```python
from build123d import *

# Parameters (mm, degrees)
F0_W     = 76
F0_H     = 46
F0_R     = 2.7
F1_DEPTH = 2
F2_R     = 6
F5_DEPTH = 25


with BuildPart() as f1:
    # F0 (on Top) → F1 (new body)
    with BuildSketch(Plane.XY):
        with Locations((-38, 0)):
            Rectangle(F0_W, F0_H)
        Polygon((-71.8, 11.2694276696), (-71.8, 15.2), (-61.6, 15.2), (-51.4, 15.2), (-51.4, 11.2694276696), (-51.4, -11.2694276696), (-51.4, -15.2), (-61.6, -15.2), (-71.8, -15.2), (-71.8, -11.2694276696), align=None, mode=Mode.SUBTRACT)
        Polygon((-50.6, 11.2694276696), (-50.6, 15.2), (-40.4, 15.2), (-30.2, 15.2), (-30.2, 11.2694276696), (-30.2, -11.2694276696), (-30.2, -15.2), (-40.4, -15.2), (-50.6, -15.2), (-50.6, -11.2694276696), align=None, mode=Mode.SUBTRACT)
        with Locations((-25.5, -6)):
            Circle(F0_R, mode=Mode.SUBTRACT)
        Polygon((-10.6, 15.2), (-0.4, 15.2), (-0.4, 11.2694276696), (-0.4, -11.2694276696), (-0.4, -15.2), (-10.6, -15.2), (-20.8, -15.2), (-20.8, -11.2694276696), (-20.8, 11.2694276696), (-20.8, 15.2), align=None, mode=Mode.SUBTRACT)
        with Locations((-25.5, 6)):
            Circle(F0_R, mode=Mode.SUBTRACT)
        with BuildLine():
            Line((-61.6, 15.2), (-71.8, 15.2))
            Line((-71.8, 15.2), (-71.8, 11.2694276696))
            ThreePointArc((-71.8, 11.2694276696), (-67.0655603291, 14.1833582162), (-61.6, 15.2))
        make_face()
        with BuildLine():
            Line((-51.4, 15.2), (-61.6, 15.2))
            ThreePointArc((-61.6, 15.2), (-56.1344396709, 14.1833582162), (-51.4, 11.2694276696))
            Line((-51.4, 11.2694276696), (-51.4, 15.2))
        make_face()
        with BuildLine():
            Line((-51.4, -15.2), (-51.4, -11.2694276696))
            ThreePointArc((-51.4, -11.2694276696), (-56.1344396709, -14.1833582162), (-61.6, -15.2))
            Line((-61.6, -15.2), (-51.4, -15.2))
        make_face()
        with BuildLine():
            ThreePointArc((-61.6, -15.2), (-67.0655603291, -14.1833582162), (-71.8, -11.2694276696))
            Line((-71.8, -11.2694276696), (-71.8, -15.2))
            Line((-71.8, -15.2), (-61.6, -15.2))
        make_face()
        with BuildLine():
            Line((-40.4, 15.2), (-50.6, 15.2))
            Line((-50.6, 15.2), (-50.6, 11.2694276696))
            ThreePointArc((-50.6, 11.2694276696), (-45.8655603291, 14.1833582162), (-40.4, 15.2))
        make_face()
        with BuildLine():
            Line((-30.2, 15.2), (-40.4, 15.2))
            ThreePointArc((-40.4, 15.2), (-34.9344396709, 14.1833582162), (-30.2, 11.2694276696))
            Line((-30.2, 11.2694276696), (-30.2, 15.2))
        make_face()
        with BuildLine():
            ThreePointArc((-20.8, 11.2694276696), (-16.0655603291, 14.1833582162), (-10.6, 15.2))
            Line((-10.6, 15.2), (-20.8, 15.2))
            Line((-20.8, 15.2), (-20.8, 11.2694276696))
        make_face()
        with BuildLine():
            Line((-0.4, 11.2694276696), (-0.4, 15.2))
            Line((-0.4, 15.2), (-10.6, 15.2))
            ThreePointArc((-10.6, 15.2), (-5.1344396709, 14.1833582162), (-0.4, 11.2694276696))
        make_face()
        with BuildLine():
            Line((-0.4, -15.2), (-0.4, -11.2694276696))
            ThreePointArc((-0.4, -11.2694276696), (-5.1344396709, -14.1833582162), (-10.6, -15.2))
            Line((-10.6, -15.2), (-0.4, -15.2))
        make_face()
        with BuildLine():
            ThreePointArc((-10.6, -15.2), (-16.0655603291, -14.1833582162), (-20.8, -11.2694276696))
            Line((-20.8, -11.2694276696), (-20.8, -15.2))
            Line((-20.8, -15.2), (-10.6, -15.2))
        make_face()
        with BuildLine():
            Line((-30.2, -15.2), (-30.2, -11.2694276696))
            ThreePointArc((-30.2, -11.2694276696), (-34.9344396709, -14.1833582162), (-40.4, -15.2))
            Line((-40.4, -15.2), (-30.2, -15.2))
        make_face()
        with BuildLine():
            ThreePointArc((-40.4, -15.2), (-45.8655603291, -14.1833582162), (-50.6, -11.2694276696))
            Line((-50.6, -11.2694276696), (-50.6, -15.2))
            Line((-50.6, -15.2), (-40.4, -15.2))
        make_face()
    extrude(amount=F1_DEPTH)

    # F2
    f2_edges = [f1.edges().sort_by_distance(p)[0] for p in [
        (-71.8, 11.269428, 1),
        (-71.8, -11.269428, 1),
        (-51.4, -11.269428, 1),
        (-51.4, 11.269428, 1),
        (-50.6, 11.269428, 1),
        (-50.6, -11.269428, 1),
        (-20.8, 11.269428, 1),
        (-20.8, -11.269428, 1),
        (-0.4, 11.269428, 1),
        (-0.4, -11.269428, 1),
        (-30.2, -11.269428, 1),
        (-30.2, 11.269428, 1),
    ]]
    fillet(f2_edges, radius=F2_R)

    # F3: F1 across face


with BuildPart() as f1_1:
    add(f1.part)
    add(f1.part.mirror(Plane(origin=(0, 0, 1), x_dir=(0, 1, 0), z_dir=(1, 0, 0))))

    # F4 (on face) → F5 (cut)
    with BuildSketch(Plane.XY.offset(2)):
        with BuildLine():
            ThreePointArc((0.4, 8.1853527719), (0, 7.7853527719), (-0.4, 8.1853527719))
            Line((-0.4, 8.1853527719), (-0.4, -8.1853527719))
            ThreePointArc((-0.4, -8.1853527719), (0, -7.7853527719), (0.4, -8.1853527719))
            Line((0.4, -8.1853527719), (0.4, 8.1853527719))
        make_face()
        with BuildLine():
            ThreePointArc((51.4, 8.1853527719), (51, 7.7853527719), (50.6, 8.1853527719))
            Line((50.6, 8.1853527719), (50.6, -8.1853527719))
            ThreePointArc((50.6, -8.1853527719), (51, -7.7853527719), (51.4, -8.1853527719))
            Line((51.4, -8.1853527719), (51.4, 8.1853527719))
        make_face()
        with BuildLine():
            ThreePointArc((-50.6, 8.1853527719), (-51, 7.7853527719), (-51.4, 8.1853527719))
            Line((-51.4, 8.1853527719), (-51.4, -8.1853527719))
            ThreePointArc((-51.4, -8.1853527719), (-51, -7.7853527719), (-50.6, -8.1853527719))
            Line((-50.6, -8.1853527719), (-50.6, 8.1853527719))
        make_face()
    extrude(amount=-F5_DEPTH, mode=Mode.SUBTRACT)


solid = f1_1.part
```
The model under review builds one solid part; all positions refer to its coordinate system, in mm. Coordinates: 2 decimals unless noted, no trailing zeros. Write each loop counter-clockwise with the first axis right and the second up, starting at its lowest first coordinate (ties: lowest second). Pieces come first, ordered by that corner, then holes. Notation, with made-up numbers: (79, -5.75) - (123, -5.75) arc R22 cw to (123, 18.25) - close; hole circle Ø5 at (76, 21.5). An arc over 180 degrees is marked (long way). Answer in a Markdown table with one row per item. Add a question column.
Q1. Consider section C-C on x = 61. Give the boundary of the cut face in (y, z), then the cut area to 3 significant figures.
Q2. Consider section A-A on x = 25.5. Give the boundary of the cut face in (y, z), then the cut area to 3 significant figures.
Q3. Consider section B-B on y = -10. Give the boundary of the cut face in (x, z), then the cut area to 3 significant figures.
Q4. Clearance check with a flat-ended pin moving along its axis: pin 1 (5 mm diameter, centred on x = -25.5, y = -6, fed in from -Z). State where the tip first meets the part, or that it passes through.
Q5. Consider section D-D on z = 0.4. Give the number of separate pieces and of enclosed holes in the cut face, then the cut area to 3 significant figures.
Q6. To check wall thickness, follow line 1 along Y through (x, z) = (25.5, 1.1); line 2 along Y through (x, z) = (10, 1.65); line 3 along X through (y, z) = (-5, 1.2). State the ranges of each line that lie inside material, in increasing order. Write a range as from..to.
Answers below:
| question | item | result |
|---|---|---|
| 1 | outline | (-23, 0) - (-15.19, 0) - (-15.19, 2) - (-23, 2) - close; (15.19, 0) - (23, 0) - (23, 2) - (15.19, 2) - close |
| 1 | area | 31.2 mm² |
| 2 | outline | (-23, 0) - (-8.7, 0) - (-8.7, 2) - (-23, 2) - close; (-3.3, 0) - (3.3, 0) - (3.3, 2) - (-3.3, 2) - close; (8.7, 0) - (23, 0) - (23, 2) - (8.7, 2) - close |
| 2 | area | 70.4 mm² |
| 3 | outline | (-76, 0) - (-71.52, 0) - (-71.52, 2) - (-76, 2) - close; (-51.68, 0) - (-50.32, 0) - (-50.32, 2) - (-51.68, 2) - close; (-30.48, 0) - (-20.52, 0) - (-20.52, 2) - (-30.48, 2) - close; (-0.68, 0) - (0.68, 0) - (0.68, 2) - (-0.68, 2) - close; (20.52, 0) - (30.48, 0) - (30.48, 2) - (20.52, 2) - close; (50.32, 0) - (51.68, 0) - (51.68, 2) - (50.32, 2) - close; (71.52, 0) - (76, 0) - (76, 2) - (71.52, 2) - close |
| 3 | area | 65.9 mm² |
| 4 | pin 1 | through |
| 5 | separate pieces | 1 |
| 5 | enclosed holes | 7 |
| 5 | area | 3,480 mm² |
| 6 | line 1 | -23..-8.7, -3.3..3.3, 8.7..23 |
| 6 | line 2 | -23..-15.19, 15.19..23 |
| 6 | line 3 | -76..-71.8, -30.2..-28.01, -22.99..-20.8, 20.8..22.99, 28.01..30.2, 71.8..76 |
